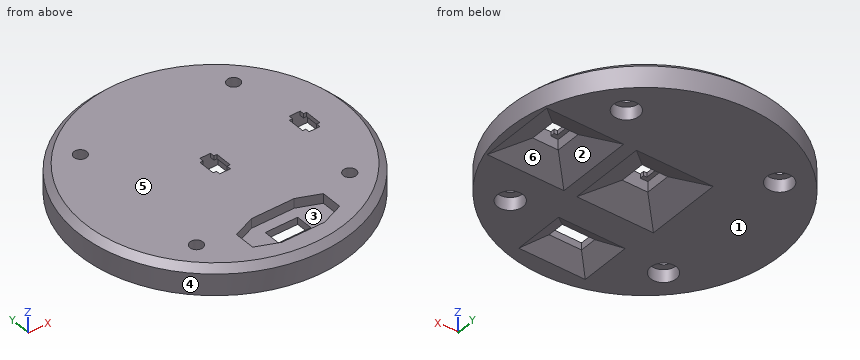
```python
from build123d import *

# Parameters (mm, degrees)
SKETCH2_R           = 31.85
BOSS_EXTRUDE1_DEPTH = 6.5
SKETCH3_W           = 6
SKETCH3_H           = 6
CUT_EXTRUDE1_DEPTH  = 6.5
CHAMFER1_SIZE       = 6
CHAMFER1_SIZE2      = 3.057152697
SKETCH5_R           = 1.5
CUT_EXTRUDE2_DEPTH  = 56.252556502
SKETCH6_R           = 3
CUT_EXTRUDE3_DEPTH  = 3
CHAMFER3_SIZE       = 1.5
BOSS_EXTRUDE2_DEPTH = 1
SKETCH10_W          = 7.6
SKETCH10_H          = 4
CUT_EXTRUDE5_DEPTH  = 46.509284767
CUT_EXTRUDE6_DEPTH  = 2.25
CHAMFER4_SIZE       = 4
CHAMFER4_SIZE2      = 2.597630373


with BuildPart() as part:
    # Sketch2 → Boss-Extrude1 (new body)
    with BuildSketch(Plane.XY.offset(-25.5)):
        Circle(SKETCH2_R)
    extrude(amount=-BOSS_EXTRUDE1_DEPTH)

    # Sketch3 → Cut-Extrude1 (cut)
    with BuildSketch(Plane(origin=(0, 0, -32), x_dir=(-1, 0, 0), z_dir=(0, 0, -1))):
        with Locations((-21, 0)):
            Rectangle(SKETCH3_W, SKETCH3_H)
        Rectangle(SKETCH3_W, SKETCH3_H)
    extrude(amount=-CUT_EXTRUDE1_DEPTH, mode=Mode.SUBTRACT)

    # Chamfer1
    chamfer1_edges = [part.edges().sort_by_distance(p)[0] for p in [
        (3, 0, -32),
        (0, -3, -32),
        (-3, 0, -32),
        (0, 3, -32),
        (24, 0, -32),
        (21, -3, -32),
        (18, 0, -32),
        (21, 3, -32),
    ]]
    chamfer1_side = [part.faces().sort_by_distance(p)[0] for p in [
        (-30.949145961, 0, -32),
    ]]
    chamfer(chamfer1_edges, length=CHAMFER1_SIZE, length2=CHAMFER1_SIZE2, reference=chamfer1_side[0])

    # Sketch5 → Cut-Extrude2 (cut, through all)
    with BuildSketch(Plane.XY):
        with Locations((-17.971861544, -17.500238124)):
            Circle(SKETCH5_R)
        with Locations((17.971861544, -17.500238124)):
            Circle(SKETCH5_R)
        with Locations((17.971861544, 17.500238124)):
            Circle(SKETCH5_R)
        with Locations((-17.971861544, 17.500238124)):
            Circle(SKETCH5_R)
    extrude(amount=-CUT_EXTRUDE2_DEPTH, mode=Mode.SUBTRACT)

    # Sketch6 → Cut-Extrude3 (cut)
    with BuildSketch(Plane.XY.offset(-32)):
        with Locations((-17.971861544, -17.500238124)):
            Circle(SKETCH6_R)
        with Locations(Location((17.971861544, -17.500238124, 0), (0, 0, 180))):
            Circle(SKETCH6_R)
        with Locations((17.971861544, 17.500238124)):
            Circle(SKETCH6_R)
        with Locations(Location((-17.971861544, 17.500238124, 0), (0, 0, 180))):
            Circle(SKETCH6_R)
    extrude(amount=CUT_EXTRUDE3_DEPTH, mode=Mode.SUBTRACT)

    # Chamfer3
    chamfer3_edges = [part.edges().sort_by_distance(p)[0] for p in [
        (-31.85, 0, -25.5),
    ]]
    chamfer(chamfer3_edges, length=CHAMFER3_SIZE)

    # Sketch7 → Boss-Extrude2 (add)
    with BuildSketch(Plane.XY.offset(-25.5)):
        Polygon((-1.25, -2), (-2, -2), (-2, 2), (-1.25, 2), (-1.25, 3), (-3, 3), (-3, -3), (-1.25, -3), align=None)
        Polygon((1.2909118, -3), (3, -3), (3, 3), (1.2909118, 3), (1.2909118, 2), (2, 2), (2, -2), (1.2909118, -2), align=None)
        Polygon((19.75, -2), (19, -2), (19, 2), (19.75, 2), (19.75, 3), (18, 3), (18, -3), (19.75, -3), align=None)
        Polygon((22.2909118, -3), (24, -3), (24, 3), (22.2909118, 3), (22.2909118, 2), (23, 2), (23, -2), (22.2909118, -2), align=None)
    extrude(amount=-BOSS_EXTRUDE2_DEPTH)

    # Sketch10 → Cut-Extrude5 (cut, through all)
    with BuildSketch(Plane(origin=(0, 0, -32), x_dir=(-1, 0, 0), z_dir=(0, 0, -1))):
        with Locations((-0.006825443, -22.003067008)):
            Rectangle(SKETCH10_W, SKETCH10_H)
    extrude(amount=-CUT_EXTRUDE5_DEPTH, mode=Mode.SUBTRACT)

    # Sketch11 → Cut-Extrude6 (cut)
    with BuildSketch(Plane.XY.offset(-25.5)):
        Polygon((-4.993522574, -17.422135009), (5.007173461, -17.422135009), (10.193224733, -19.552209326), (10.193224733, -24.45392469), (5.007173461, -26.583999007), (-4.993522574, -26.583999007), (-10.179573846, -24.45392469), (-10.179573846, -19.552209326), align=None)
    extrude(amount=-CUT_EXTRUDE6_DEPTH, mode=Mode.SUBTRACT)

    # Chamfer4
    chamfer4_edges = [part.edges().sort_by_distance(p)[0] for p in [
        (-3.793174557, -22.003067008, -32),
        (0.006825443, -20.003067008, -32),
        (3.806825443, -22.003067008, -32),
        (0.006825443, -24.003067008, -32),
    ]]
    chamfer4_side = [part.faces().sort_by_distance(p)[0] for p in [
        (-30.949145961, 0, -32),
    ]]
    chamfer(chamfer4_edges, length=CHAMFER4_SIZE, length2=CHAMFER4_SIZE2, reference=chamfer4_side[0])


solid = part.part
```
For this review, take the finished solid that the model builds, in its own axes (mm). Face numbers are marked on the shaded views. A direction names the side the tool comes from. Give positions to 0.01 mm unless a question says otherwise; leave off trailing zeros. Write each loop counter-clockwise with the first axis right and the second up, starting at its lowest first coordinate (ties: lowest second). Pieces come first, ordered by that corner, then holes.
Item 1: Insertion check: P1, Ø1.4, axis at x = 2, y = 0, coming from the -Z side; P2, Ø10, axis at x = 12.5, y = -3.5, coming from the -Z side; P3, Ø2, axis at x = 6.5, z = -28.5, coming from the -Y side; P4, Ø0.5, axis at y = 0, z = -26, coming from the -X side. Each pin has a flat end and moves straight along its axis. Give the tip position at first contact, or say it passes through.
Item 2: Machinability: for the marked faces 1, 2 and 3, which of the approach directions +Z, -Z, +X, -X, +Y, -Y give a long, thin tool a straight path to every point of the face, cutting with its end or side? Answer none if there is none.
Item 3: Take a section at A-A (y = 0). Give the boundary of the cut face in (x, z).
Item 4: The part is to be moulded in two halves that separate along X. For the marked faces 4, 5 and 6, say which applies: +X half, -X half, draft (parallel to the pull), parting line (faces both ways), or undercut.
Item 5: Take a section at B-B (x = 0). Give the boundary of the cut face in (y, z).
Item 6: Wall thickness on probe 1 along X at (y, z) = (-4.5, -30); probe 2 along Y at (x, z) = (-17, -30.5); probe 3 along Y at (x, z) = (-1.5, -30.5): over which ranges is each line inside the solid? List them lowest first.
Established:
1. P1: stops at z = -26.5
1. P2: stops at z = -32
1. P3: stops at y = -31.37
1. P4: stops at x = -31.1
2. face 1: -Z, +X, -X, +Y, -Y
2. face 2: -Z
2. face 3: +Z
3. outline: (-31.85, -32) - (-9, -32) - (-3, -28.94) - (-3, -26.5) - (-2, -26.5) - (-2, -25.5) - (-30.35, -25.5) - (-31.85, -27) - close; (2, -26.5) - (3, -26.5) - (3, -28.94) - (9, -32) - (12, -32) - (18, -28.94) - (18, -26.5) - (19, -26.5) - (19, -25.5) - (2, -25.5) - close; (23, -26.5) - (24, -26.5) - (24, -28.94) - (30, -32) - (31.85, -32) - (31.85, -27) - (30.35, -25.5) - (23, -25.5) - close
4. face 4: parting line
4. face 5: draft
4. face 6: undercut
5. outline: (-31.85, -32) - (-28, -32) - (-24, -29.4) - (-24, -27.75) - (-26.58, -27.75) - (-26.58, -25.5) - (-30.35, -25.5) - (-31.85, -27) - close; (-20, -29.4) - (-16, -32) - (-9, -32) - (-3, -28.94) - (-3, -25.5) - (-17.42, -25.5) - (-17.42, -27.75) - (-20, -27.75) - close; (3, -28.94) - (9, -32) - (31.85, -32) - (31.85, -27) - (30.35, -25.5) - (3, -25.5) - close
6. probe 1: x = -31.53 to -5.07, 5.07 to 15.93, 26.07 to 31.53
6. probe 2: y = -26.93 to -20.34, -14.66 to 14.66, 20.34 to 26.93
6. probe 3: y = -31.81 to -25.69, -18.31 to -6.06, 6.06 to 31.81
